Geometry check sheet. Reference: the model listing, model coordinates, mm. A direction names the side the tool comes from. Coordinates: 2 decimals unless noted, no trailing zeros. Put each result on its own line as item: value. Start each with the question number.
from build123d import *

# Parameters (mm, degrees)
F3_R = 1.5
F4_R = 5


# Not quite as in the source:
# - a fillet or chamfer that OpenCascade refuses, or shapes differently, is made with other operations: its cross-section is extruded or revolved along the edge and cut away or added


with BuildPart() as f1:
    # F0 (on Front) → F1 (revolve)
    with BuildSketch(Plane.XZ):
        with BuildLine():
            Line((-3.2761832158, -65.334129345), (-5.337398374, -62.834129345))
            ThreePointArc((-5.337398374, -62.834129345), (-6.7311516997, -51.7224852161), (-12.8360642807, -42.334129345))
            Line((-12.8360642807, -42.334129345), (-13.4396579748, -38.334129345))
            ThreePointArc((-13.4396579748, -38.334129345), (-12.3713927582, -35.334129345), (-13.4396579748, -32.334129345))
            Line((-13.4396579748, -32.334129345), (-14.137398374, 4.665870655))
            Line((-14.137398374, 4.665870655), (-15.637398374, 4.665870655))
            Line((-15.637398374, 4.665870655), (-16.837398374, -50.334129345))
            ThreePointArc((-16.837398374, -50.334129345), (-9.9295742391, -59.4637716742), (-6.337398374, -70.334129345))
            Line((-6.337398374, -70.334129345), (-6.337398374, -75.334129345))
            Line((-6.337398374, -75.334129345), (-0.337398374, -75.334129345))
            Line((-0.337398374, -75.334129345), (-0.337398374, -65.334129345))
            Line((-0.337398374, -65.334129345), (-3.2761832158, -65.334129345))
        make_face()
    revolve(axis=Axis((-19.837398374, 0, -35.334129345), (0, 0, 1)))

    # F2: fillet of radius 3 on 1 edges, made by hand

    # F2_s1 → F2_t2 (revolve, cut)
    with BuildSketch(Plane.XZ):
        with BuildLine():
            ThreePointArc((-0.336998374, -68.3344507591), (-1.1942035822, -66.2342669991), (-3.2761749277, -65.3337294309))
            Line((-3.2761749277, -65.3337294309), (-3.2699560145, -65.0336572981))
            ThreePointArc((-3.2699560145, -65.0336572981), (-1.8067866508, -65.0339927765), (-0.337398374, -65.0339927765))
            Line((-0.337398374, -65.0339927765), (-0.0372618054, -65.334129345))
            ThreePointArc((-0.0372618054, -65.334129345), (-0.0372618054, -66.8342900521), (-0.0368618054, -68.3344507591))
            Line((-0.0368618054, -68.3344507591), (-0.336998374, -68.3344507591))
        make_face()
    revolve(axis=Axis((-19.837398374, 0, -65.334129345), (0, 0, 1)), mode=Mode.SUBTRACT)

    # F3
    f3_edges = [f1.edges().sort_by_distance(p)[0] for p in [
        (-33.337398, 0, -75.334129),
        (-39.337398, 0, -75.334129),
    ]]
    fillet(f3_edges, radius=F3_R)

    # F4
    f4_edges = [f1.edges().sort_by_distance(p)[0] for p in [
        (-22.837398, 0, -50.334129),
    ]]
    fillet(f4_edges, radius=F4_R)


solid = f1.part
Item 1: Mould release check, pull along X, two halves, no side actions. Record for faces 3 (the conical face through (-20.624, 5.993, -13.575)), 4 (the conical face through (-16.498, -1.385, -22.141)), 5 (the cylindrical face through (-7.367, -5.171, -72.109)), 6 (the flat face through (-22, -4, 4.666)): released by +X, released by -X, zero draft, split by the parting line, or undercut.
Item 2: Scan lines: line 1 along Y through (x, z) = (-14, -57); line 2 along X through (y, z) = (5, -43.5); line 3 along X through (y, z) = (0, 1.5). Record each from-to range of solid material in increasing order. Write a range as [from, to].
Item 3: Access from +Z, -Z, +X, -X, +Y, -Y to the whole of each face (thin tool, end or side, straight path). Record for faces 1 (the conical face through (-13.58, 1.97, -39.42)), 2 (the flat face through (-16, 15, -75.334)).
Item 4: Go/stop test with flat-tipped pins: P1, Ø12, axis at y = -13.5, z = -47, coming from the -X side; P2, Ø2, axis at x = -30, z = -60, coming from the -Y side; P3, Ø21.5, axis at x = -19.84, y = 0, coming from the -Z side. Record where each tip stops, or that it passes through.
From the geometry:
1. face 3: split by the parting line
1. face 4: undercut
1. face 5: undercut
1. face 6: zero draft
2. line 1: [-13.17, -6.16], [6.16, 13.17]
2. line 2: [-26.25, -13.42]
2. line 3: [-25.6, -23.97], [-15.71, -14.08]
3. face 1: none
3. face 2: -Z, +X, -X, +Y, -Y
4. P1: x = -29.06
4. P2: y = -11.4
4. P3: z = -61.19
